The model under review builds one solid part; all positions refer to its coordinate system, in mm. Round coordinates to 2 decimals unless told otherwise and drop trailing zeros. Order: outer loops, then holes, each group sorted by start corner. A loop starts at its lowest first (then second) coordinate and runs counter-clockwise, first axis right, second up.
```python
from build123d import *

# Parameters (mm, degrees)
PAD_DEPTH     = 1.7
SKETCH001_W   = 37.9
SKETCH001_H   = 4
SKETCH001_W_2 = 10.4
SKETCH001_H_2 = 1
POCKET_DEPTH  = 1.701
FILLET_R      = 1
FILLET002_R   = 2
FILLET003_R   = 0.99
SKETCH002_R   = 0.6
HOLE_DEPTH    = 25


with BuildPart() as part:
    # Sketch → Pad (new body)
    with BuildSketch(Plane.XY):
        Polygon((0, 0), (100, 0), (100, 25), (75, 25), (75, 55), (0, 55), align=None)
    extrude(amount=-PAD_DEPTH)

    # Sketch001 → Pocket (cut, through all)
    with BuildSketch(Plane.XY):
        with Locations((67.45, 2)):
            Rectangle(SKETCH001_W, SKETCH001_H)
        with Locations((94.8, 0.5)):
            Rectangle(SKETCH001_W_2, SKETCH001_H_2)
    extrude(amount=-POCKET_DEPTH, mode=Mode.SUBTRACT)

    # Fillet
    fillet_edges = [part.edges().sort_by_distance(p)[0] for p in [
        (48.5, 4, -0.85),
        (86.4, 4, -0.85),
    ]]
    fillet(fillet_edges, radius=FILLET_R)

    # Fillet002
    fillet002_edges = [part.edges().sort_by_distance(p)[0] for p in [
        (75, 55, -0.85),
        (75, 25, -0.85),
    ]]
    fillet(fillet002_edges, radius=FILLET002_R)

    # Fillet003
    fillet003_edges = [part.edges().sort_by_distance(p)[0] for p in [
        (89.6, 1, -0.85),
    ]]
    fillet(fillet003_edges, radius=FILLET003_R)

    # Sketch002 → Hole (cut)
    with BuildSketch(Plane.XY):
        with Locations((88, 1.4)):
            Circle(SKETCH002_R)
        with Locations((88, 8)):
            Circle(SKETCH002_R)
    extrude(amount=-HOLE_DEPTH, mode=Mode.SUBTRACT)


solid = part.part
```
(1) Consider section A-A (z = -0.75). State how many separate pieces and enclosed holes the cut face has, and give its area (3 significant figures).
Data:
separate pieces: 1
enclosed holes: 2
area: 4,590 mm2
(2) To check wall thickness, follow probe 1 along Y at (x, z) = (88, -0.4); probe 2 along X at (y, z) = (3, -1); probe 3 along X at (y, z) = (36, -0.3). State the ranges of each line that lie inside material, in increasing order.
Data:
probe 1: y = 0 to 0.8, 2 to 7.4, 8.6 to 25
probe 2: x = 0 to 48.5, 86.4 to 100
probe 3: x = 0 to 75
(3) Insertion check: pin 1 (0.5 mm diameter, centred on x = 93.5, z = -1, fed in from -Y); pin 2 (0.5 mm diameter, centred on x = 65, z = -0.5, fed in from -Y); pin 3 (0.8 mm diameter, centred on x = 90.5, z = -0.5, fed in from +Y); pin 4 (1.1 mm diameter, centred on x = 88, y = 8, fed in from -Z). Each pin has a flat end and moves straight along its axis. Give the tip position at first contact, or say it passes through.
Data:
pin 1: stops at y = 1
pin 2: stops at y = 4
pin 3: stops at y = 25
pin 4: passes through
(4) Consider section C-C (y = 34). Write out the cut boundary in (x, z), and give its area (4 significant figures).
Data:
outline: (0, -1.7) - (75, -1.7) - (75, 0) - (0, 0) - close
area: 127.5 mm2
(5) Draft analysis for pull direction Z (two halves, no side actions). For faces 1 (the flat face through (38, 28, 0)), 2 (the flat face through (38, 28, -1.7)), 3 (the cylindrical face through (74.43, 54.4, -0.86)), state which applies: pulls with the +Z half, pulls with the -Z half, needs draft (parallel to the pull), parting line crosses it, or undercut.
Data:
face 1: pulls with the +Z half
face 2: pulls with the -Z half
face 3: needs draft
(6) Consider section B-B (x = 70). Write out the cut boundary in (y, z).
Data:
outline: (4, -1.7) - (55, -1.7) - (55, 0) - (4, 0) - close
